```python
from build123d import *

# Parameters (mm, degrees)
BOSS_EXTRUDE1_DEPTH                  = 25.4
F_35_64_0_54688_DIAMETER_HOLE1_D     = 13.890752
F_35_64_0_54688_DIAMETER_HOLE1_DEPTH = 35.052
F_35_64_0_54688_DIAMETER_HOLE1_TIP   = 4.173202923
F_10_32_TAPPED_HOLE1_D               = 4.0386
F_10_32_TAPPED_HOLE1_DEPTH           = 8.636
F_10_32_TAPPED_HOLE1_TIP             = 1.213317848
FILLET1_R                            = 6.35


with BuildPart() as part:
    # Sketch1 → Boss-Extrude1 (new body)
    with BuildSketch(Plane.XY):
        Polygon((0, 0), (61.591726717, 0), (61.591726717, -15.24), (86.991726717, -15.24), (86.991726717, 0), (148.583453434, 0), (86.991726717, 35.56), (61.591726717, 35.56), align=None)
    extrude(amount=BOSS_EXTRUDE1_DEPTH)

    # 35/64 (0.54688) Diameter Hole1
    with Locations(Plane(origin=(0, 35.56, 0), x_dir=(1, 0, 0), z_dir=(0, 1, 0))):
        with Locations((74.291726717, -12.7)):
            Hole(F_35_64_0_54688_DIAMETER_HOLE1_D / 2, depth=F_35_64_0_54688_DIAMETER_HOLE1_DEPTH)
            with Locations((0, 0, -(F_35_64_0_54688_DIAMETER_HOLE1_DEPTH + F_35_64_0_54688_DIAMETER_HOLE1_TIP / 2))):  # 118° drill point
                Cone(0, F_35_64_0_54688_DIAMETER_HOLE1_D / 2, F_35_64_0_54688_DIAMETER_HOLE1_TIP, mode=Mode.SUBTRACT)

    # #10-32 Tapped Hole1
    with Locations(Plane(origin=(0, -15.24, 0), x_dir=(-1, 0, 0), z_dir=(0, -1, 0))):
        with Locations((-77.466726717, -15.875), (-71.116726717, -9.525)):
            Hole(F_10_32_TAPPED_HOLE1_D / 2, depth=F_10_32_TAPPED_HOLE1_DEPTH)
            with Locations((0, 0, -(F_10_32_TAPPED_HOLE1_DEPTH + F_10_32_TAPPED_HOLE1_TIP / 2))):  # 118° drill point
                Cone(0, F_10_32_TAPPED_HOLE1_D / 2, F_10_32_TAPPED_HOLE1_TIP, mode=Mode.SUBTRACT)

    # Fillet1
    fillet1_edges = [part.edges().sort_by_distance(p)[0] for p in [
        (86.991726717, 0, 12.7),
        (61.591726717, 0, 12.7),
    ]]
    fillet(fillet1_edges, radius=FILLET1_R)


solid = part.part
```
Work out the finished part from the listing and answer in its coordinate system (mm). A direction names the side the tool comes from. Give positions to 0.01 mm unless a question says otherwise; leave off trailing zeros. Write each loop counter-clockwise with the first axis right and the second up, starting at its lowest first coordinate (ties: lowest second). Pieces come first, ordered by that corner, then holes.
(1) The part is cut by section C-C on x = 102. Write down the section's boundary in (y, z), plus the area to 3 significant figures.
Final values:
outline: (0, 0) - (26.89, 0) - (26.89, 25.4) - (0, 25.4) - close
area: 683 mm2
(2) The part is cut by section D-D on x = 132. Write down the section's boundary in (y, z), plus the area to 3 significant figures.
Final values:
outline: (0, 0) - (9.57, 0) - (9.57, 25.4) - (0, 25.4) - close
area: 243 mm2
(3) The mould has two halves that part along Z. Classify faces 1 (the cylindrical face through (75.45, -10.86, 15.79)), 2 (the flat face through (69, 35.56, 7)), 3 (the flat face through (73, 11, 0)): pulls with the +Z half, pulls with the -Z half, needs draft (parallel to the pull), parting line crosses it, or undercut.
Final values:
face 1: undercut
face 2: needs draft
face 3: pulls with the -Z half
(4) Straight lines are drawn through the part: line 1 (X direction, y = 4.5, z = 17.25); line 2 (X direction, y = 15, z = 6.5); line 3 (Y direction, x = 20, z = 1.75). For each, find the intervals that lie inside material, in ascending order.
Final values:
line 1: x = 7.79 to 69.04, 79.54 to 140.79
line 2: x = 25.98 to 71.16, 77.42 to 122.6
line 3: y = 0 to 11.55
(5) Which of the six approach directions +Z, -Z, +X, -X, +Y, -Y give full straight-line access (tool end or side, diameter ignored) to faces 4 (the cylindrical face through (69.1, -10.9, 9.4)), 5 (the flat face through (61.592, -11, 13)), 6 (the cylindrical face through (67.67, 17.79, 10.61)), 7 (the flat face through (86.992, -11, 13))?
Final values:
face 4: -Y
face 5: +Z, -Z, -X, -Y
face 6: +Y
face 7: +Z, -Z, +X, -Y
(6) Flat-ended cylindrical pins translate along their axes: pin 1 Ø5.5 at (x, z) = (77.47, 15.88) entering from +Y; pin 2 Ø7 at (y, z) = (-10.5, 10) entering from -X; pin 3 Ø7.5 at (x, z) = (134, 7) entering from -Y; pin 4 Ø2 at (x, z) = (69, 12) entering from +Y. Find the tip coordinate at first contact, or state that the pin passes through.
Final values:
pin 1: stops at y = 35.56
pin 2: stops at x = 61.59
pin 3: stops at y = 0
pin 4: stops at y = 0.14
(7) The part is cut by section A-A on z = 23. Write down the section's boundary in (x, y), plus the area to 3 significant figures.
Final values:
outline: (0, 0) - (55.24, 0) arc R6.35 cw to (61.59, -6.35) - (61.59, -15.24) - (86.99, -15.24) - (86.99, -6.35) arc R6.35 cw to (93.34, 0) - (148.58, 0) - (86.99, 35.56) - (61.59, 35.56) - close
area: 3,500 mm2
(8) The part is cut by section B-B on y = 11. Write down the section's boundary in (x, z).
Final values:
outline: (19.05, 0) - (129.53, 0) - (129.53, 25.4) - (19.05, 25.4) - close; hole circle Ø13.89 at (74.29, 12.7)
